Design review of the part built by this model. Coordinates are the model's own, in mm. A direction names the side the tool comes from. Round coordinates to 2 decimals unless told otherwise and drop trailing zeros. Loops run counter-clockwise (first coordinate to the right, second up) from the corner with the lowest first, then second, coordinate; pieces in that order, holes last. Notation, with made-up numbers: (-26.5, 9.25) - (20.5, 9.25) arc R26 cw to (20.5, 26.25) - close; hole circle Ø3 at (11, 58.25). An arc over 180 degrees is marked (long way). Return JSON: item names as keys, results as strings. Group by question number.
(1) We need section C-C, the plane y = 72.5. Write out the cut boundary in (x, z), and give its area (3 significant figures).
(2) We need section D-D, the plane z = -28.5. Write out the cut boundary in (x, y), and give its area (3 significant figures).
(3) For faces 4 (the flat face through (56, -22.062, -7)), 5 (the flat face through (6, 0, -35)), 6 (the flat face through (60, -26, -6.64)), list the 3-axis set-ups (+Z, -Z, +X, -X, +Y, -Y) from which the entire face can be reached by the end or side of a thin tool; tool diameter is ignored.
(4) Clearance check with flat-ended pins moving along their axes: pin 1 (8 mm diameter, centred on x = 11, y = 64.5, fed in from -Z); pin 2 (21 mm diameter, centred on y = 11, z = 10.5, fed in from +X); pin 3 (4 mm diameter, centred on x = 79.5, z = -14, fed in from +Y). State where each tip first meets the part, or that it passes through.
(5) We need section A-A, the plane x = 76. Write out the cut boundary in (y, z), and give its area (3 significant figures).
(6) The part is to be moulded in two halves that separate along Z. For faces 1 (the flat face through (25, -5, 27.062)), 2 (the flat face through (60, -26, 6.64)), 3 (the flat face through (52, -30, 8)), say which applies: pulls with the +Z half, pulls with the -Z half, needs draft (parallel to the pull), parting line crosses it, or undercut.
(7) Wall thickness on L1, parallel to Y at x = 5, z = 0; L2, parallel to Z at x = 42, y = -4; L3, parallel to Y at x = 18, z = -30: over which ranges is each line inside the solid? List them lowest first. Write a range as [from, to].
(8) We need section B-B, the plane z = 0. Write out the cut boundary in (x, y), and give its area (3 significant figures).
from build123d import *

# Parameters (mm, degrees)
CROQUIS1_W              = 70
CROQUIS1_H              = 110
CROQUIS1_R              = 6.35
SALIENTE_EXTRUIR1_DEPTH = 7.9375
CROQUIS2_W              = 97.0625
CROQUIS2_H              = 70
SALIENTE_EXTRUIR2_DEPTH = 7.9375
SALIENTE_EXTRUIR3_DEPTH = 7.9375


with BuildPart() as part:
    # Croquis1 → Saliente-Extruir1 (new body)
    with BuildSketch(Plane(origin=(0, 0, 0), x_dir=(0, 0, -1), z_dir=(1, 0, 0))):
        with Locations((0, 25)):
            Rectangle(CROQUIS1_W, CROQUIS1_H)
        with Locations((0, 60.378740827)):
            Circle(CROQUIS1_R, mode=Mode.SUBTRACT)
    extrude(amount=SALIENTE_EXTRUIR1_DEPTH)

    # Croquis2 → Saliente-Extruir2 (add)
    with BuildSketch(Plane.XZ.offset(30)):
        with Locations((56.46875, 0)):
            Rectangle(CROQUIS2_W, CROQUIS2_H)
        with BuildLine():
            ThreePointArc((30, -6.640349162), (23.359650838, 0), (30, 6.640349162))
            Line((30, 6.640349162), (90, 6.640349162))
            ThreePointArc((90, 6.640349162), (96.640349162, 0), (90, -6.640349162))
            Line((90, -6.640349162), (30, -6.640349162))
        make_face(mode=Mode.SUBTRACT)
    extrude(amount=-SALIENTE_EXTRUIR2_DEPTH)

    # Croquis3 → Saliente-Extruir3 (add)
    with BuildSketch(Plane(origin=(0, 0, 35), x_dir=(-1, 0, 0), z_dir=(0, 0, -1))):
        Polygon((0, 45.166428926), (-75.166428926, -30), (0, -30), align=None)
    extrude(amount=SALIENTE_EXTRUIR3_DEPTH)


solid = part.part
Solutions:
{
 "1": {"outline": "(0, -35) - (7.94, -35) - (7.94, 35) - (0, 35) - close", "area": "556 mm^2"},
 "2": {"outline": "(0, -30) - (105, -30) - (105, -22.06) - (7.94, -22.06) - (7.94, 80) - (0, 80) - close", "area": "1,640 mm^2"},
 "3": {"face 4": "-Z, +X, +Y", "face 5": "-Z, +X, -X, +Y, -Y", "face 6": "+Y, -Y"},
 "4": {"pin 1": "z = -35", "pin 2": "x = 7.94", "pin 3": "y = -22.06"},
 "5": {"outline": "(-30, -35) - (-22.06, -35) - (-22.06, -6.64) - (-30, -6.64) - close; (-30, 6.64) - (-22.06, 6.64) - (-22.06, 35) - (-30, 35) - close", "area": "450 mm^2"},
 "6": {"face 1": "pulls with the -Z half", "face 2": "undercut", "face 3": "needs draft"},
 "7": {"L1": "[-30, 54.03], [66.73, 80]", "L2": "[27.06, 35]", "L3": "[-30, -22.06]"},
 "8": {"outline": "(0, -30) - (23.36, -30) - (23.36, -22.06) - (7.94, -22.06) - (7.94, 54.03) - (0, 54.03) - close; (0, 66.73) - (7.94, 66.73) - (7.94, 80) - (0, 80) - close; (96.64, -30) - (105, -30) - (105, -22.06) - (96.64, -22.06) - close", "area": "961 mm^2"}
}
